Part model, mm, in its own coordinate system. Face numbers are marked on the shaded views. A direction names the side the tool comes from. Coordinates: 2 decimals unless noted, no trailing zeros. Loops run counter-clockwise (first coordinate to the right, second up) from the corner with the lowest first, then second, coordinate; pieces in that order, holes last. Notation, with made-up numbers: (-22, 18.25) - (-11, 18.25) arc R10 ccw to (-11, 22.25) - close; hole circle Ø1 at (84.25, 7.5). An arc over 180 degrees is marked (long way). One line per question, with ' | ' between items. Start each with the question number.
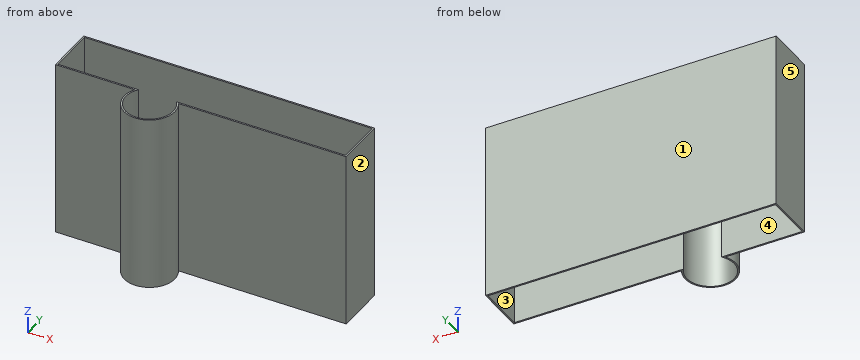
Autodesk Inventor part; units mm, degrees
ref_plane "YZ Plane" through (0, 0, 0) normal (1, 0, 0) x (0, 1, 0)
ref_plane "XZ Plane" through (0, 0, 0) normal (0, 1, 0) x (-1, 0, 0)
ref_plane "XY Plane" through (0, 0, 0) normal (0, 0, 1) x (1, 0, 0)
sketch "Sketch1" plane through (0, 0, 0) normal (0, 0, 1) x (1, 0, 0)
  line L0 (584.2, 0) -> (584.2, 101.6)
  line L1 (584.2, 101.6) -> (0, 101.6)
  line L2 (0, 101.6) -> (0, 0)
  line L3 (0, 0) -> (159.2059, 0)
  line L4 (247.1941, 0) -> (584.2, 0)
  arc A0 (159.2059, 0) -> (247.1941, 0) centre (203.2, -25.4) ccw
  dimension "d2" = 101.6
  dimension "d4" = 203.2
  dimension "d5" = 50.8
  dimension "d6" = 25.4
  dimension "d8" = 584.2
extrude "Extrusion1" add sketch "Sketch1" along normal blind 355.6
shell "Shell1" thickness 3.175 removed faces 2 at (277.1314, 67.7333, 0) at (277.1314, 67.7333, 355.6)
properties part number "LauncherMockup"
1) Band-saw the part on B-B on y = -25.4. List the corners of the cut face in (x, z) (3 decimals).
2) Pin check, flat tip, straight feed: pin 1 Ø4 at (x, z) = (376.5, 292) entering from -Y. Stop position of the tip, or through.
3) Tool access for the marked faces 4 and 5: list every direction of +Z, -Z, +X, -X, +Y, -Y with a clear straight run to the whole face (end or side of a thin tool).
4) Band-saw the part on C-C on z = 142. List the corners of the cut face in (x, y) (3 decimals), then the cut area to 3 significant figures.
5) Wall check: line 1 along Y through (x, z) = (149, 297.5) (3 decimals); line 2 along X through (y, z) = (75, 114) (3 decimals); line 3 along X through (y, z) = (-25.4, 224.5) (3 decimals). Give the ranges that are in metal, low to high. Write a range as [from, to].
6) Mould opens along Y. For the marked faces 1, 2 and 3 say: +Y half, -Y half, draft (parallel to the pull), parting line (faces both ways), or undercut.
7) Band-saw the part on A-A on x = 139.5. List the corners of the cut face in (y, z) (3 decimals), then the cut area to 3 significant figures.
Values found:
1) outline: (152.4, 0) - (155.575, 0) - (155.575, 355.6) - (152.4, 355.6) - close; (250.825, 0) - (254, 0) - (254, 355.6) - (250.825, 355.6) - close
2) pin 1: y = 0
3) face 4: +Z, -Z | face 5: +Z, -Z, -X, +Y, -Y
4) outline: (0, 0) - (159.206, 0) arc R50.8 ccw (long way) to (247.194, 0) - (584.2, 0) - (584.2, 101.6) - (0, 101.6) - close; hole (3.175, 3.175) - (165.1, 3.175) arc R47.625 ccw (long way) to (241.3, 3.175) - (581.025, 3.175) - (581.025, 98.425) - (3.175, 98.425) - close | area: 4,730 mm²
5) line 1: [0, 3.175], [98.425, 101.6] | line 2: [0, 3.175], [581.025, 584.2] | line 3: [152.4, 155.575], [250.825, 254]
6) face 1: +Y half | face 2: draft | face 3: undercut
7) outline: (0, 0) - (3.175, 0) - (3.175, 355.6) - (0, 355.6) - close; (98.425, 0) - (101.6, 0) - (101.6, 355.6) - (98.425, 355.6) - close | area: 2,260 mm²
